```python
from build123d import *

# Parameters (mm, degrees)
PAD046_DEPTH = 8
PAD045_DEPTH = 8
BOX008_W     = 14
BOX008_H     = 27
BOX008_DEPTH = 15.5


with BuildPart() as obj1:
    # Sketch047 → Pad046 (new body)
    with BuildSketch(Plane(origin=(0, 19, 4), x_dir=(1, 0, 0), z_dir=(0, 1, 0))):
        Polygon((-6, 3.5), (6, 3.5), (6, -3.5), (3.5, -3.5), (3.5, -4.5), (1.75, -4.5), (1.75, -5.5), (-1.75, -5.5), (-1.75, -4.5), (-3.5, -4.5), (-3.5, -3.5), (-6, -3.5), align=None)
    extrude(amount=PAD046_DEPTH)


with BuildPart() as obj2:
    # Sketch046 → Pad045 (new body)
    with BuildSketch(Plane(origin=(0, 0, 0), x_dir=(-1, 0, 0), z_dir=(0, 1, 0))):
        Polygon((-6, 3.5), (6, 3.5), (6, -3.5), (3.5, -3.5), (3.5, -4.5), (1.75, -4.5), (1.75, -5.5), (-1.75, -5.5), (-1.75, -4.5), (-3.5, -4.5), (-3.5, -3.5), (-6, -3.5), align=None)
    extrude(amount=PAD045_DEPTH)


with BuildPart() as obj3:
    # Box008 → Box008 (new body)
    with BuildSketch(Plane(origin=(-7, 0, -5.8), x_dir=(1, 0, 0), z_dir=(0, 0, 1))):
        with Locations((7, 13.5)):
            Rectangle(BOX008_W, BOX008_H)
    extrude(amount=BOX008_DEPTH)

    # Cut015: cut obj2
    add(obj2.part, mode=Mode.SUBTRACT)

    # Cut016: cut obj1
    add(obj1.part, mode=Mode.SUBTRACT)


solid = obj3.part
```
Could you check a few things on this model? Use its own coordinates, in mm. A direction names the side the tool comes from. Coordinates: 2 decimals unless noted, no trailing zeros. Order: outer loops, then holes, each group sorted by start corner. A loop starts at its lowest first (then second) coordinate and runs counter-clockwise, first axis right, second up. Notation, with made-up numbers: M -37.75,-34 L -24.75,-34 A33 cw -24.75,-1 Z; hole C -26,-22.75 d9. An arc over 180 degrees is marked long. Use one line per item in the form item = value. Start each with the question number.
1. Suppose I cut it at D-D on x = -4. Write out the boundary of the cut face in (y, z).
2. On a 3-axis mill with a long thin cutter (end or side, diameter ignored), from which of +Z, -Z, +X, -X, +Y, -Y can I reach the whole of each face in a straight line? I mean faces 5 (the flat face through (-3.5, 4, -4)), 6 (the flat face through (3, 23, 8.5)), 7 (the flat face through (0, 14, -5.8)). Say none if no direction works.
3. We'd pull the mould along X, two halves only. Please class faces 1 (the flat face through (6, 4, 0)), 2 (the flat face through (6, 23, 4)), 3 (the flat face through (-7, 13, 2)), 4 (the flat face through (0, 14, 9.7)): +X half, -X half, draft (parallel to the pull), parting line (faces both ways), or undercut.
4. Please list where these lines run through material, in increasing order: line 1 (Z direction, x = -2.75, y = 22.25); line 2 (X direction, y = 24.5, z = 7); line 3 (Z direction, x = 5.5, y = 3.5).
5. Suppose I cut it at C-C on x = 0.75. Write out the boundary of the cut face in (y, z), then the cut area to 4 significant figures.
6. Suppose I cut it at B-B on z = 5. Write out the boundary of the cut face in (x, y), then the cut area to 3 significant figures.
7. Suppose I cut it at A-A on y = 22.75. Write out the boundary of the cut face in (x, z), then the cut area to 4 significant figures.
Geometry says:
q1.outline = M 0,-5.8 L 27,-5.8 L 27,0.5 L 19,0.5 L 19,7.5 L 27,7.5 L 27,9.7 L 0,9.7 L 0,3.5 L 8,3.5 L 8,-3.5 L 0,-3.5 Z
q2.face_5 = -Y
q2.face_6 = +Y
q2.face_7 = -Z, +X, -X, +Y, -Y
q3.face_1 = undercut
q3.face_2 = undercut
q3.face_3 = -X half
q3.face_4 = draft
q4.line_1 = -5.8 to 0.5, 8.5 to 9.7
q4.line_2 = -7 to -6, 6 to 7
q4.line_3 = -5.8 to -3.5, 3.5 to 9.7
q5.outline = M 0,-5.8 L 27,-5.8 L 27,0.5 L 19,0.5 L 19,9.5 L 27,9.5 L 27,9.7 L 0,9.7 L 0,3.5 L 8,3.5 L 8,-5.5 L 0,-5.5 Z
q5.area = 274.5 mm^2
q6.outline = M -7,0 L 7,0 L 7,27 L 6,27 L 6,19 L -6,19 L -6,27 L -7,27 Z
q6.area = 282 mm^2
q7.outline = M -7,-5.8 L 7,-5.8 L 7,9.7 L -7,9.7 Z; hole M -6,0.5 L 6,0.5 L 6,7.5 L 3.5,7.5 L 3.5,8.5 L 1.75,8.5 L 1.75,9.5 L -1.75,9.5 L -1.75,8.5 L -3.5,8.5 L -3.5,7.5 L -6,7.5 Z
q7.area = 122.5 mm^2
